The model under review builds one solid part; all positions refer to its coordinate system, in mm. A direction names the side the tool comes from. Coordinates: 2 decimals unless noted, no trailing zeros. Loops run counter-clockwise (first coordinate to the right, second up) from the corner with the lowest first, then second, coordinate; pieces in that order, holes last. Notation, with made-up numbers: (21.25, 52) - (62.25, 52) arc R13 cw to (62.25, 57) - close; hole circle Ø6 at (59, -3.5). An arc over 180 degrees is marked (long way). Answer in a Markdown table with one row per item. Add a question column.
(1) For line 1 along X through (y, z) = (-833, 2912); line 2 along Y through (x, z) = (-641.5, 3533); line 3 along Y through (x, z) = (-624, 3747), list the stretches that pass through material, from the lowest coordinate up.
(2) Machinability: for faces 1 (the cylindrical face through (-180.68, -107.94, 3933.1)), 2 (the cylindrical face through (-1207.2, -567.2, 3184.1)), 3 (the flat face through (-908.37, -37.9, 3860.55)), 4 (the cylindrical face through (-603.4, -567.2, 3184.1)), which of the approach directions +Z, -Z, +X, -X, +Y, -Y give a long, thin tool a straight path to every point of the face, cutting with its end or side? Answer none if there is none.
(3) We need section C-C on y = -509.5. Write out the cut boundary in (x, z), plus the area to 3 significant figures.
(4) We need section B-B on z = 3674. Write out the cut boundary in (x, y), plus the area to 3 significant figures.
(5) We need section D-D on x = -227. Write out the cut boundary in (y, z).
(6) For P1, Ø15, axis at y = -585, z = 3210.5, coming from the -X side; P2, Ø12, axis at x = -1147, y = -1032.5, coming from the -Z side; P3, Ø6, axis at x = -1198, y = -832.5, coming from the +Z side, all flat-tipped, find the tip position at first contact; note any pin that passes through.
(7) We need section A-A on x = -865.5. Write out the cut boundary in (y, z).
(8) Mouldability with a two-part tool opening along Z and no side actions: class faces 5 (the cylindrical face through (-206.033, -582.195, 3184.105)), 6 (the cylindrical face through (-1682.45, -84.55, 3944.07)), 7 (the flat face through (-588.633, -543, 3193)), 8 (the flat face through (-424.32, -37.9, 3860.55)) as +Z half, -Z half, draft (parallel to the pull), parting line (faces both ways), or undercut.
from build123d import *

# Parameters (mm, degrees)
CROQUIS1_W              = 1500
CROQUIS1_H              = 1910
CROQUIS1_W_2            = 1300
CROQUIS1_H_2            = 1695.501409597
SALIENTE_EXTRUIR1_DEPTH = 100
CROQUIS2_W              = 50
CROQUIS2_H              = 100
SALIENTE_EXTRUIR2_DEPTH = 110
CROQUIS3_R              = 27.184499999
SALIENTE_EXTRUIR3_DEPTH = 55
REDONDEO1_R             = 50
REDONDEO2_R             = 110
REDONDEO3_R             = 40
SIMETR_A6_START         = -205.332665454
SIMETR_A6_DEPTH         = 50
SIMETR_A6_2_OUTLINE_R   = 27.184499999
SIMETR_A6_2_DEPTH       = 105
CROQUIS4_W              = 100
CROQUIS4_H              = 1695.501409597
SALIENTE_EXTRUIR4_DEPTH = 100
CROQUIS5_R              = 25
CORTAR_EXTRUIR1_DEPTH   = 30
CROQUIS6_R              = 25
CORTAR_EXTRUIR3_DEPTH   = 4447.028443617


with BuildPart() as part:
    # Croquis1 → Saliente-Extruir1 (new body)
    with BuildSketch(Plane(origin=(0, -1955.253607577, 1610.989797583), x_dir=(1, 0, 0), z_dir=(0, 0.771778946447621, -0.6358909166045701))):
        with Locations((-905.332665454, -2110.391476147)):
            Rectangle(CROQUIS1_W, CROQUIS1_H)
        with Locations((-905.332665454, -2107.640771349)):
            Rectangle(CROQUIS1_W_2, CROQUIS1_H_2, mode=Mode.SUBTRACT)
    extrude(amount=SALIENTE_EXTRUIR1_DEPTH)

    # Croquis2 → Saliente-Extruir2 (add)
    with BuildSketch(Plane(origin=(0, 1949.254595519, 2365.804603911), x_dir=(1, 0, 0), z_dir=(-5.363902149474557e-15, 0.6358909166045701, 0.771778946447621))):
        with Locations((-1630.332665455, -2583.437348319)):
            Rectangle(CROQUIS2_W, CROQUIS2_H)
    extrude(amount=-SALIENTE_EXTRUIR2_DEPTH)

    # Croquis3 → Saliente-Extruir3 (add)
    with BuildSketch(Plane.ZY.offset(1655.332665454)):
        with Locations(Location((3970.000000001, -76.38250521, 0), (0, 0, 180))):
            Circle(CROQUIS3_R)
    extrude(amount=SALIENTE_EXTRUIR3_DEPTH)

    # Redondeo1
    redondeo1_edges = [part.edges().sort_by_distance(p)[0] for p in [
        (-1630.332665454, -83.176906702, 4040.383493154),
    ]]
    fillet(redondeo1_edges, radius=REDONDEO1_R)

    # Redondeo2
    # the kernel refuses this fillet: 110 mm, written as the material it takes off along each edge
    with BuildSketch(Plane(origin=(-1360.383691176, -153.124907529, 3955.487809045), x_dir=(-5.363902149475724e-15, 0.6358909166045759, 0.7717789464476161), z_dir=(-1, 0, 0))) as redondeo2_piece_1:
        with BuildLine():
            CenterArc((110, 97.979589711), REDONDEO2_R, 180, 62.964308211)
            Line((0, 97.979589711), (0, 0))
            Line((0, 0), (60, 0))
        make_face()
    extrude(amount=539.897948557, mode=Mode.SUBTRACT)

    # Redondeo3
    redondeo3_edges = [part.edges().sort_by_distance(p)[0] for p in [
        (-1630.332665454, -114.971452533, 4001.794545831),
    ]]
    fillet(redondeo3_edges, radius=REDONDEO3_R)

    # Simetría6: read off the stored shape, not the designer's step
    # Simetría6 outline → Simetría6 (add)
    with BuildSketch(Plane.YZ.offset(SIMETR_A6_START)):
        with BuildLine():
            ThreePointArc((-117.519718806, 3980.993137388), (-107.655684266, 3932.466465304), (-77.506323008, 3893.183477935))
            Line((-77.506323008, 3893.183477935), (-75.947012884, 3891.898717384))
            Line((-75.947012884, 3891.898717384), (-5.999012058, 3976.794401493))
            Line((-5.999012058, 3976.794401493), (-44.58795938, 4008.588947324))
            ThreePointArc((-44.58795938, 4008.588947324), (-62.233936584, 4017.956417776), (-82.138761146, 4019.667549947))
            ThreePointArc((-82.138761146, 4019.667549947), (-107.046738875, 4006.933211198), (-117.519718806, 3980.993137388))
        make_face()
    extrude(amount=SIMETR_A6_DEPTH)

    # Simetr_a6 2 outline → Simetr_a6 2 (add)
    with BuildSketch(Plane.YZ.offset(SIMETR_A6_START)):
        with Locations((-76.38250521, 3970.000000001)):
            Circle(SIMETR_A6_2_OUTLINE_R)
    extrude(amount=SIMETR_A6_2_DEPTH)

    # Croquis4 → Saliente-Extruir4 (add)
    with BuildSketch(Plane(origin=(0, -1878.075712932, 1547.400705922), x_dir=(1, 0, 0), z_dir=(0, 0.771778946447621, -0.63589091660457))):
        with Locations((-1172.032665454, -2107.640771349)):
            Rectangle(CROQUIS4_W, CROQUIS4_H)
        with Locations((-638.632665454, -2107.640771349)):
            Rectangle(CROQUIS4_W, CROQUIS4_H)
    extrude(amount=-SALIENTE_EXTRUIR4_DEPTH)

    # Croquis5 → Cortar-Extruir1 (cut)
    with BuildSketch(Plane(origin=(-588.632665454, 0, 0), x_dir=(0, 0, -1), z_dir=(1, 0, 0))):
        with Locations((-3207.950961806, -574.685890092)):
            Circle(CROQUIS5_R)
    cortar_extruir1 = extrude(amount=-CORTAR_EXTRUIR1_DEPTH, mode=Mode.SUBTRACT)

    # Croquis6 → Cortar-Extruir3 (cut, through all)
    with BuildSketch(Plane.ZY.offset(255.332665454)):
        with Locations(Location((3207.950961806, -574.685890092, 0), (0, 0, 180))):
            Circle(CROQUIS6_R)
    cortar_extruir3 = extrude(amount=-CORTAR_EXTRUIR3_DEPTH, mode=Mode.SUBTRACT)

    # Simetría11: Cortar-Extruir1, Cortar-Extruir3 across plane
    add(cortar_extruir1.mirror(Plane(origin=(-905.332665454, 0, 0), x_dir=(0, 0, 1), z_dir=(1, 0, 0))), mode=Mode.SUBTRACT)
    add(cortar_extruir3.mirror(Plane(origin=(-905.332665454, 0, 0), x_dir=(0, 0, 1), z_dir=(1, 0, 0))), mode=Mode.SUBTRACT)


solid = part.part
Outcome:
| question | item | result |
|---|---|---|
| 1 | line 1 | -1655.33 to -1555.33, -1222.03 to -1122.03, -688.63 to -588.63, -255.33 to -155.33 |
| 1 | line 2 | -371.65 to -242.08 |
| 1 | line 3 | -195.33 to -65.76 |
| 2 | face 1 | +X, -X, -Y |
| 2 | face 2 | -X |
| 2 | face 3 | -Z, -Y |
| 2 | face 4 | +X |
| 3 | outline | (-1655.33, 3208.44) - (-1555.33, 3208.44) - (-1555.33, 3365.7) - (-1655.33, 3365.7) - close; (-1222.03, 3208.44) - (-1122.03, 3208.44) - (-1122.03, 3365.7) - (-1222.03, 3365.7) - close; (-688.63, 3208.44) - (-588.63, 3208.44) - (-588.63, 3365.7) - (-688.63, 3365.7) - close; (-255.33, 3208.44) - (-155.33, 3208.44) - (-155.33, 3365.7) - (-255.33, 3365.7) - close |
| 3 | area | 62,900 mm² |
| 4 | outline | (-1655.33, -255.48) - (-1555.33, -255.48) - (-1555.33, -125.91) - (-1655.33, -125.91) - close; (-1222.03, -255.48) - (-1122.03, -255.48) - (-1122.03, -125.91) - (-1222.03, -125.91) - close; (-688.63, -255.48) - (-588.63, -255.48) - (-588.63, -125.91) - (-688.63, -125.91) - close; (-255.33, -255.48) - (-155.33, -255.48) - (-155.33, -125.91) - (-255.33, -125.91) - close |
| 4 | area | 51,800 mm² |
| 5 | outline | (-1220.55, 2502.7) - (-1143.37, 2439.11) - (71.18, 3913.21) - (-6, 3976.79) - close; hole circle Ø50 at (-574.69, 3207.95) |
| 6 | P1 | x = -1192.03 |
| 6 | P2 | z = 2566.39 |
| 6 | P3 | z = 2977.31 |
| 7 | outline | (-1220.55, 2502.7) - (-1143.37, 2439.11) - (-1076.92, 2519.76) - (-1154.1, 2583.35) - close; (-75.95, 3891.9) - (1.23, 3828.31) - (71.18, 3913.21) - (-6, 3976.79) - close |
| 8 | face 5 | undercut |
| 8 | face 6 | parting line |
| 8 | face 7 | draft |
| 8 | face 8 | -Z half |
